Can you work these out from the drawing? Everything is in mm from the part's minimum corner. A direction names the side the tool comes from. Coordinates: 2 decimals unless noted, no trailing zeros. Order: outer loops, then holes, each group sorted by start corner. A loop starts at its lowest first (then second) coordinate and runs counter-clockwise, first axis right, second up. Notation, with made-up numbers: (3, 14) - (47, 14) arc R11 cw to (47, 22) - close; hole circle Ø1 at (47, -3). An arc over 180 degrees is marked (long way). One line per item, written item: value.
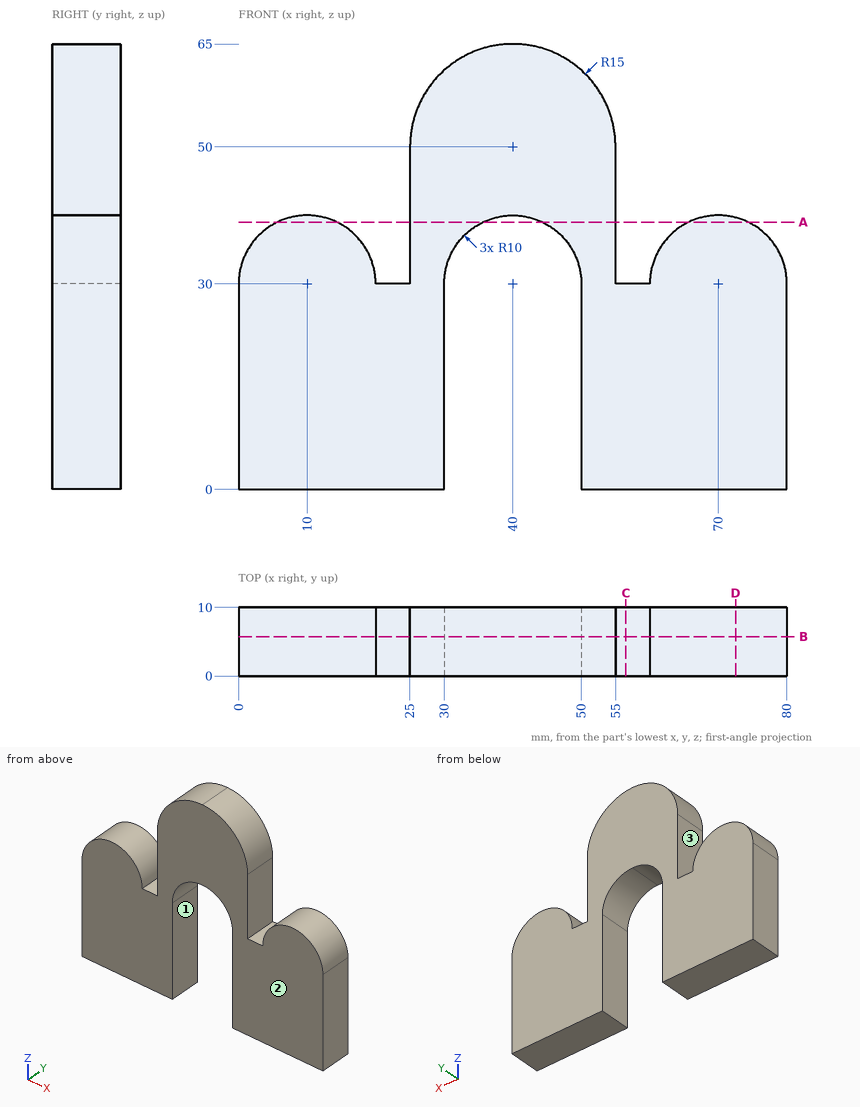
Item 1: For the marked faces 1, 2 and 3, which set-ups out of +Z, -Z, +X, -X, +Y, -Y let a thin tool reach every point of the face, with its end or its side?
Conclusion:
face 1: -Z, +Y, -Y
face 2: +Z, -Z, +X, -X, -Y
face 3: +Z, +Y, -Y
Item 2: I'm going to push flat-ended pins straight in: pin 1 Ø1.5 at (x, y) = (21.5, 4.5) entering from +Z; pin 2 Ø3 at (y, z) = (6, 44) entering from -X; pin 3 Ø4 at (y, z) = (5, 39) entering from -X; pin 4 Ø6 at (x, z) = (29.5, 57.5) entering from -Y. Where does each tip first touch, or does it pass through?
Conclusion:
pin 1: z = 30
pin 2: x = 25
pin 3: x = 2.86
pin 4: y = 0
Item 3: I want a section at A-A on z = 39. Please give me the cut outline in (x, y).
Conclusion:
outline: (5.64, 0) - (14.36, 0) - (14.36, 10) - (5.64, 10) - close; (25, 0) - (35.64, 0) - (35.64, 10) - (25, 10) - close; (44.36, 0) - (55, 0) - (55, 10) - (44.36, 10) - close; (65.64, 0) - (74.36, 0) - (74.36, 10) - (65.64, 10) - close
Item 4: If I drill on probe 1 along X at (y, z) = (8.5, 16.5); probe 2 along X at (y, z) = (1, 31); probe 3 along X at (y, z) = (6.5, 43), over which ranges is the centre line in solid material (lowest first)?
Conclusion:
probe 1: 0 to 30, 50 to 80
probe 2: 0.05 to 19.95, 25 to 30.05, 49.95 to 55, 60.05 to 79.95
probe 3: 25 to 55
Item 5: I want a section at C-C on x = 56.5. Please give me the cut outline in (y, z), then the cut area to 3 significant figures.
Conclusion:
outline: (0, 0) - (10, 0) - (10, 30) - (0, 30) - close
area: 300 mm²
Item 6: I want a section at B-B on y = 5.75. Please give me the cut outline in (x, z).
Conclusion:
outline: (0, 0) - (30, 0) - (30, 30) arc R10 cw to (40, 40) arc R10 cw to (50, 30) - (50, 0) - (80, 0) - (80, 30) arc R10 ccw to (60, 30) - (55, 30) - (55, 50) arc R15 ccw to (40, 65) arc R15 ccw to (25, 50) - (25, 30) - (20, 30) arc R10 ccw to (0, 30) - close
Item 7: I want a section at D-D on x = 72.5. Please give me the cut outline in (y, z).
Conclusion:
outline: (0, 0) - (10, 0) - (10, 39.68) - (0, 39.68) - close
